The model under review builds one solid part; all positions refer to its coordinate system, in mm. A direction names the side the tool comes from. Coordinates: 2 decimals unless noted, no trailing zeros. Write each loop counter-clockwise with the first axis right and the second up, starting at its lowest first coordinate (ties: lowest second). Pieces come first, ordered by that corner, then holes. Notation, with made-up numbers: M 57.5,-34 L 98.5,-34 A15 cw 98.5,-5 Z; hole C 8.25,-5.5 d3. An arc over 180 degrees is marked long. Answer as a JSON object with one key per item and string values.
```python
from build123d import *

# Parameters (mm, degrees)
BOSS_EXTRUDE1_DEPTH      = 5
BOSS_EXTRUDE1_DEPTH_BACK = 5
SKETCH3_W                = 1.15
SKETCH3_H                = 8.4


with BuildPart() as part:
    # Sketch1 → Boss-Extrude1 (new, two sides: drawn at the far end of the back side and taken through both)
    with BuildSketch(Plane(origin=(0, 0, 0), x_dir=(0, 0, -1), z_dir=(1, 0, 0)).offset(-BOSS_EXTRUDE1_DEPTH_BACK)):
        with BuildLine():
            Line((9.5, -14.09787218), (9.5, 14.09787218))
            ThreePointArc((9.5, 14.09787218), (0, 17), (-9.5, 14.09787218))
            Line((-9.5, 14.09787218), (-9.5, -14.09787218))
            ThreePointArc((-9.5, -14.09787218), (0, -17), (9.5, -14.09787218))
        make_face()
    extrude(amount=BOSS_EXTRUDE1_DEPTH + BOSS_EXTRUDE1_DEPTH_BACK)

    # Sketch2 → Cut-Revolve1 (revolve, cut)
    with BuildSketch(Plane.XY, mode=Mode.PRIVATE) as cut_revolve1_sk:
        Polygon((-5, 0), (-5, 6), (-3, 6), (-3, 8), (5, 8), (5, 0), align=None)
    revolve(cut_revolve1_sk.sketch.rotate(Axis((5, 0, 0), (-1, 0, 0)), 180), axis=Axis((5, 0, 0), (-1, 0, 0)), mode=Mode.SUBTRACT)

    # Sketch3 → Cut-Revolve2 (revolve, cut)
    with BuildSketch(Plane.XY, mode=Mode.PRIVATE) as cut_revolve2_sk:
        with Locations((2.575, 4.2)):
            Rectangle(SKETCH3_W, SKETCH3_H)
    revolve(cut_revolve2_sk.sketch.rotate(Axis((3.15, 0, 0), (-1, 0, 0)), 180), axis=Axis((3.15, 0, 0), (-1, 0, 0)), mode=Mode.SUBTRACT)

    # Sketch4 → Cut-Revolve3 (revolve, cut)
    with BuildSketch(Plane.XY, mode=Mode.PRIVATE) as cut_revolve3_sk:
        Polygon((-5, -12.5), (-5, -10), (-4.567, -10.433), (4.567, -10.433), (5, -10), (5, -12.5), align=None)
    revolve(cut_revolve3_sk.sketch.rotate(Axis((5, -12.5, 0), (-1, 0, 0)), 270), axis=Axis((5, -12.5, 0), (-1, 0, 0)), mode=Mode.SUBTRACT)

    # Sketch5 → Cut-Revolve4 (revolve, cut)
    with BuildSketch(Plane.XY, mode=Mode.PRIVATE) as cut_revolve4_sk:
        Polygon((-5, 12.5), (-5, 15), (-4.567, 14.567), (4.567, 14.567), (5, 15), (5, 12.5), align=None)
    revolve(cut_revolve4_sk.sketch.rotate(Axis((5, 12.5, 0), (-1, 0, 0)), 270), axis=Axis((5, 12.5, 0), (-1, 0, 0)), mode=Mode.SUBTRACT)


solid = part.part
```
(1) Add section B-B on x = -0.75. Give the boundary of the cut face in (y, z).
Results list:
{"outline": "M -14.1,-9.5 L 14.1,-9.5 A17 ccw 14.1,9.5 L -14.1,9.5 A17 ccw Z; hole C -12.5,0 d4.13; hole C 0,0 d16; hole C 12.5,0 d4.13"}
(2) For pin 1 Ø6 at (x, z) = (-3.5, -5.5) entering from +Y; pin 2 Ø2 at (x, z) = (0.5, -6) entering from +Y; pin 3 Ø2 at (x, z) = (-1.5, -5) entering from +Y, all flat-tipped, find the tip position at first contact; note any pin that passes through.
Results list:
{"pin 1": "y = 16.82", "pin 2": "y = 16.25", "pin 3": "y = 16.52"}
(3) Wall thickness on line 1 along Z through (x, y) = (-2, 0); line 2 along X through (y, z) = (-7, 1.5); line 3 along Z through (x, y) = (-4.5, 0): over which ranges is each line inside the solid? List them lowest first. Write a range as from..to.
Results list:
{"line 1": "-9.5..-8, 8..9.5", "line 2": "-5..-3", "line 3": "-9.5..-6, 6..9.5"}
(4) Draft analysis for pull direction X (two halves, no side actions). For faces 1 (the face through (2.583, -8.012, 2.523)), 2 (the face through (-3, -2, 6)), 3 (the face through (0, -17, 0)), state which applies: released by +X, released by -X, zero draft, split by the parting line, or undercut.
Results list:
{"face 1": "undercut", "face 2": "released by +X", "face 3": "zero draft"}
(5) Add section D-D on x = -4. Give the boundary of the cut face in (y, z).
Results list:
{"outline": "M -14.1,-9.5 L 14.1,-9.5 A17 ccw 14.1,9.5 L -14.1,9.5 A17 ccw Z; hole C -12.5,0 d4.13; hole C 0,0 d12; hole C 12.5,0 d4.13"}
(6) Add section A-A on y = -12.5. Give the boundary of the cut face in (x, z).
Results list:
{"outline": "M -5,-9.5 L 5,-9.5 L 5,-2.5 L 4.57,-2.07 L -4.57,-2.07 L -5,-2.5 Z; M -5,2.5 L -4.57,2.07 L 4.57,2.07 L 5,2.5 L 5,9.5 L -5,9.5 Z"}
(7) Add section C-C on z = 5. Give the boundary of the cut face in (x, y) (3 decimals), and give its area (3 significant figures).
Results list:
{"outline": "M -5,-16.248 L 5,-16.248 L 5,-6.245 L 3.15,-6.245 L 3.15,-6.75 L 2,-6.75 L 2,-6.245 L -3,-6.245 L -3,-3.317 L -5,-3.317 Z; M -5,3.317 L -3,3.317 L -3,6.245 L 2,6.245 L 2,6.75 L 3.15,6.75 L 3.15,6.245 L 5,6.245 L 5,16.248 L -5,16.248 Z", "area": "211 mm²"}
(8) For faces 4 (the face through (-0.46, 1.73, -7.81)), 5 (the face through (-5, 0.2, 6.5)), list the 3-axis set-ups (+Z, -Z, +X, -X, +Y, -Y) from which the entire face can be reached by the end or side of a thin tool; tool diameter is ignored.
Results list:
{"face 4": "+X", "face 5": "+Z, -Z, -X, +Y, -Y"}
